The drawing under review shows one solid part. Ordinate dimensions are in mm from its lowest x, y, z. A direction names the side the tool comes from. Coordinates: 2 decimals unless noted, no trailing zeros. Write each loop counter-clockwise with the first axis right and the second up, starting at its lowest first coordinate (ties: lowest second). Pieces come first, ordered by that corner, then holes. Notation, with made-up numbers: M 64.5,13.25 L 88.5,13.25 A17 cw 88.5,43.25 Z; hole C 71,-36 d9. An arc over 180 degrees is marked long. Write item = value, one per line.
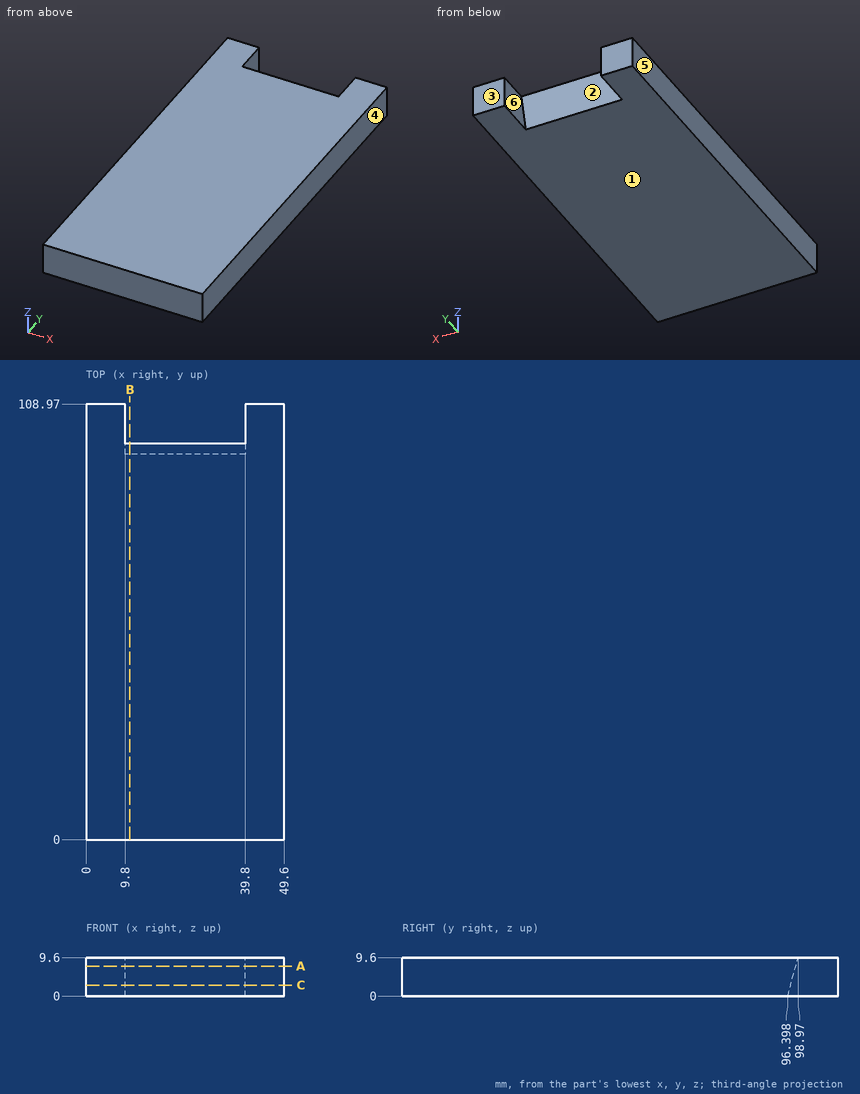
Q1. The part is to be moulded in two halves that separate along X. For the marked faces 3, 4, 5 and 6, say which applies: +X half, -X half, draft (parallel to the pull), parting line (faces both ways), or undercut.
Check result:
face_3 = draft
face_4 = +X half
face_5 = -X half
face_6 = undercut
Q2. Wall thickness on line 1 (X direction, y = 102.5, z = 7.75); line 2 (Y direction, x = 25, z = 7.75) (1 decimal); line 3 (Y direction, x = 22, z = 6.25): over which ranges is each line inside the solid? List them lowest first.
Check result:
line_1 = 0 to 9.8, 39.8 to 49.6
line_2 = 0 to 98.5
line_3 = 0 to 98.07
Q3. Consider section B-B, the plane x = 11. State the section outline as (y, z) points, and give its area (3 significant figures).
Check result:
outline = M 0,0 L 96.4,0 L 98.97,9.6 L 0,9.6 Z
area = 938 mm²
Q4. Consider section C-C, the plane z = 2.75. State the section outline as (x, y) points (1 decimal), and give its area (3 significant figures).
Check result:
outline = M 0,0 L 49.6,0 L 49.6,109 L 39.8,109 L 39.8,97.1 L 9.8,97.1 L 9.8,109 L 0,109 Z
area = 5,050 mm²
Q5. Consider section A-A, the plane z = 7.5. State the section outline as (x, y) points, and give its area (3 significant figures).
Check result:
outline = M 0,0 L 49.6,0 L 49.6,108.97 L 39.8,108.97 L 39.8,98.41 L 9.8,98.41 L 9.8,108.97 L 0,108.97 Z
area = 5,090 mm²
Q6. Machinability: for the marked faces 1 and 2, which of the approach directions +Z, -Z, +X, -X, +Y, -Y give a long, thin tool a straight path to every point of the face, cutting with its end or side? Answer none if there is none.
Check result:
face_1 = -Z, +X, -X, +Y, -Y
face_2 = -Z, +Y
